CAD build for the part. Positions are in the model's coordinates, mm. Face numbers are marked on the shaded views. A direction names the side the tool comes from. Coordinates: 2 decimals unless noted, no trailing zeros. Loops run counter-clockwise (first coordinate to the right, second up) from the corner with the lowest first, then second, coordinate; pieces in that order, holes last.
1) Saw through at A-A, the plane z = -27. Write the cut outline in (x, y), and give its area (3 significant figures).
2) Which spindle directions (+Z, -Z, +X, -X, +Y, -Y) get a long thin tool onto all of the face, cutting with end or side? Do the marked faces 5 and 6. Say none if no direction does.
3) Saw through at B-B, the plane y = 5.5. Write the cut outline in (x, z) (3 decimals), and give its area (3 significant figures).
4) Saw through at D-D, the plane x = -42. Write the cut outline in (y, z).
5) Wall check: line 1 along X through (y, z) = (2, -112); line 2 along X through (y, z) = (31.1, 0); line 3 along Z through (x, y) = (-31.5, 1.7). Give the ranges that are in metal, low to high.
6) Pin check, flat tips, straight feed: pin 1 Ø7.5 at (x, z) = (31.5, 112) entering from +Y; pin 2 Ø10 at (y, z) = (14.5, -15.5) entering from -X; pin 3 Ø16 at (y, z) = (17.5, -48) entering from +X (3 decimals). Stop position of each tip, or through.
7) Saw through at C-C, the plane x = -31.5. Write the cut outline in (y, z).
8) Two-plate mould, pull along Y, no slides. Class the marked faces 1, 2, 3 and 4: +Y half, -Y half, draft (parallel to the pull), parting line (faces both ways), or undercut.
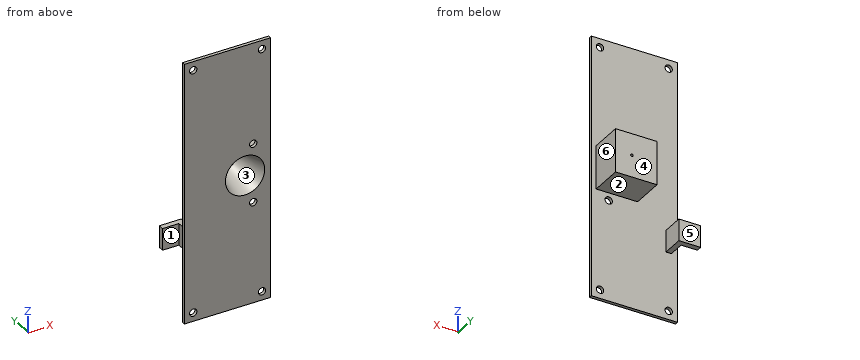
Autodesk Inventor part; units mm, degrees
ref_plane "YZ Plane" through (0, 0, 0) normal (1, 0, 0) x (0, 1, 0)
ref_plane "XZ Plane" through (0, 0, 0) normal (0, 1, 0) x (-1, 0, 0)
ref_plane "XY Plane" through (0, 0, 0) normal (0, 0, 1) x (1, 0, 0)
sketch "Sketch44" plane through (0, 0, 0) normal (0, 1, 0) x (-1, 0, 0)
  line L0 (-39.5, 120) -> (39.5, 120)
  line L1 (39.5, 120) -> (39.5, -120)
  line L2 (39.5, -120) -> (-39.5, -120)
  line L3 (-39.5, -120) -> (-39.5, 120)
  line L4 (-39.5, 120) -> (39.5, -120) construction
  line L5 (39.5, 120) -> (-39.5, -120) construction
  point P0 (0, 0)
  dimension "d138" = 79
  dimension "d139" = 240
extrude "Extrusion33" add sketch "Sketch44" along normal blind 3
sketch "Sketch45" plane through (0, 3, 0) normal (0, 1, 0) x (1, 0, 0)
  line L0 (35, -20) -> (-3, -20)
  line L1 (-3, -20) -> (-3, 20)
  line L2 (-3, 20) -> (35, 20)
  line L3 (35, 20) -> (35, -20)
  point P0 (0, 0)
  dimension "d142" = 38
  dimension "d143" = 40
extrude "Extrusion34" add sketch "Sketch45" along normal blind 30
sketch "Sketch47" plane through (0, 0, 0) normal (0, -1, 0) x (1, 0, 0)
  circle A0 centre (16, 0) radius 18
  point P0 (0, 0)
  dimension "d146" = 36
extrude "Extrusion35" cut sketch "Sketch47" against normal blind 30 draft -15
sketch "Sketch60" plane through (0, 3, 0) normal (0, 1, 0) x (1, 0, 0)
  line L0 (-33.965, 38.3247) -> (-28.965, 38.3247)
  line L1 (-28.965, 38.3247) -> (-28.965, 58.3247)
  line L2 (-28.965, 58.3247) -> (-33.965, 58.3247)
  line L3 (-33.965, 58.3247) -> (-33.965, 38.3247)
  point P0 (0, 0)
  dimension "d164" = 5
  dimension "d165" = 20
extrude "Extrusion40" add sketch "Sketch60" along normal blind 20
sketch "Sketch61" plane through (0, 23, 0) normal (0, 1, 0) x (1, 0, 0)
  line L0 (-28.965, 38.3247) -> (-28.965, 58.3247)
  line L1 (-28.965, 38.3247) -> (-48.965, 38.3247)
  line L2 (-48.965, 38.3247) -> (-48.965, 58.3247)
  line L3 (-48.965, 58.3247) -> (-28.965, 58.3247)
  line L4 (-28.965, 58.3247) -> (-28.965, 38.3247)
  point P0 (0, 0)
  dimension "d168" = 20
  dimension "d169" = 20
extrude "Extrusion41" add sketch "Sketch61" against normal blind 5
sketch "Sketch68" plane through (0, 3, 0) normal (0, 1, 0) x (1, 0, 0)
  circle A0 centre (-31.5, -112) radius 3.35
  circle A1 centre (31.5, -112) radius 3.35
  circle A2 centre (-31.5, 112) radius 3.35
  circle A3 centre (31.5, 112) radius 3.35
  point P0 (0, 0)
  dimension "d192" = 6.7
  dimension "d193" = 6.7
  dimension "d194" = 6.7
  dimension "d195" = 6.7
extrude "Extrusion46" cut sketch "Sketch68" against normal through all
sketch "Sketch69" plane through (0, 3, 0) normal (0, 1, 0) x (1, 0, 0)
  circle A0 centre (23.5, -27) radius 3.35
  circle A1 centre (23.5, 27) radius 3.35
  point P0 (0, 0)
  dimension "d198" = 6.7
  dimension "d199" = 6.7
extrude "Extrusion47" cut sketch "Sketch69" against normal through all
sketch "Sketch74" plane through (0, 33, 0) normal (0, 1, 0) x (1, 0, 0)
  circle A0 centre (20, 0) radius 1.15
  point P0 (0, 0)
  dimension "d210" = 2.3
extrude "Extrusion51" cut sketch "Sketch74" against normal blind 10
equation "\"d193\" = d192"
equation "\"d194\" = d192"
equation "\"d195\" = d192"
equation "\"d198\" = d192"
equation "\"d199\" = d192"
properties part number "liquid port_v12"
Data:
1. outline: (-39.5, 0) - (20.15, 0) - (20.15, 3) - (-39.5, 3) - close; (26.85, 0) - (39.5, 0) - (39.5, 3) - (26.85, 3) - close
1. area: 217 mm2
2. face 5: +Z, -Z, +X, -X, +Y
2. face 6: +Z, -Z, +X, +Y
3. outline: (-33.965, -58.325) - (-28.965, -58.325) - (-28.965, -38.325) - (-33.965, -38.325) - close; (-3, -20) - (35, -20) - (35, 20) - (-3, 20) - close; hole circle Ø33.053 at (16, 0)
3. area: 762 mm2
4. outline: (18, -58.32) - (23, -58.32) - (23, -38.32) - (18, -38.32) - close
5. line 1: x = -39.5 to -34.85, -28.15 to 28.15, 34.85 to 39.5
5. line 2: x = -3 to 18.85, 21.15 to 35
5. line 3: z = -120 to -115.35, -108.65 to 108.65, 115.35 to 120
6. pin 1: stops at y = 3
6. pin 2: stops at x = -3
6. pin 3: stops at x = -28.965
7. outline: (0, -120) - (3, -120) - (3, -115.35) - (0, -115.35) - close; (0, -108.65) - (3, -108.65) - (3, -58.32) - (23, -58.32) - (23, -38.32) - (3, -38.32) - (3, 108.65) - (0, 108.65) - close; (0, 115.35) - (3, 115.35) - (3, 120) - (0, 120) - close
8. face 1: undercut
8. face 2: draft
8. face 3: -Y half
8. face 4: +Y half
